Read the model definition and answer for the solid it produces. Units are mm, in the model's axes. A direction names the side the tool comes from. Coordinates: 2 decimals unless noted, no trailing zeros. Order: outer loops, then holes, each group sorted by start corner. A loop starts at its lowest first (then second) coordinate and runs counter-clockwise, first axis right, second up. Notation, with made-up numbers: (82.5, 85.25) -> (133.5, 85.25) arc R20 ccw to (133.5, 123.25) -> close; hole circle Ø4 at (-30.5, 59). An arc over 180 degrees is marked (long way). Use CSV: the item, a comma, the result in double quotes.
```python
from build123d import *

# Parameters (mm, degrees)
SKETCH1_R           = 10.16
BOSS_EXTRUDE1_DEPTH = 9.525
SKETCH2_W           = 20.151524415
SKETCH2_H           = 15.754496301
BOSS_EXTRUDE4_DEPTH = 3.175
BOSS_EXTRUDE5_DEPTH = 4.699
SKETCH4_W           = 11.36474419
SKETCH4_H           = 5.089940764
SKETCH4_W_2         = 11.314127359
BOSS_EXTRUDE6_DEPTH = 8.763
SKETCH5_W           = 19.083811061
SKETCH5_H           = 5.089940764
SKETCH5_W_2         = 19.185044725
BOSS_EXTRUDE7_DEPTH = 5.969


with BuildPart() as part:
    # Sketch1 → Boss-Extrude1 (new body)
    with BuildSketch(Plane.XY):
        Circle(SKETCH1_R)
    extrude(amount=-BOSS_EXTRUDE1_DEPTH)

    # Sketch2 → Boss-Extrude4 (add)
    with BuildSketch(Plane(origin=(0, 0, -9.525), x_dir=(-1, 0, 0), z_dir=(0, 0, -1))):
        with Locations((-0.084237792, 7.877248151)):
            Rectangle(SKETCH2_W, SKETCH2_H)
    extrude(amount=-BOSS_EXTRUDE4_DEPTH)

    # Sketch3 → Boss-Extrude5 (add)
    with BuildSketch(Plane(origin=(0, 15.754496301, 0), x_dir=(1, 0, 0), z_dir=(0, 1, 0))):
        Polygon((-9.991524415, 9.525), (-22.594029854, 9.525), (-22.594029854, 4.435059236), (23.166117059, 4.435059236), (23.166117059, 9.525), align=None)
    extrude(amount=BOSS_EXTRUDE5_DEPTH)

    # Sketch4 → Boss-Extrude6 (add)
    with BuildSketch(Plane(origin=(0, 20.453496301, 0), x_dir=(1, 0, 0), z_dir=(0, 1, 0))):
        with Locations((-16.911657759, 6.980029618)):
            Rectangle(SKETCH4_W, SKETCH4_H)
        with Locations((17.50905338, 6.980029618)):
            Rectangle(SKETCH4_W_2, SKETCH4_H)
    extrude(amount=BOSS_EXTRUDE6_DEPTH)

    # Sketch5 → Boss-Extrude7 (add)
    with BuildSketch(Plane(origin=(0, 29.216496301, 0), x_dir=(1, 0, 0), z_dir=(0, 1, 0))):
        with Locations((-13.052124324, 6.980029618)):
            Rectangle(SKETCH5_W, SKETCH5_H)
        with Locations((13.573594697, 6.980029618)):
            Rectangle(SKETCH5_W_2, SKETCH5_H)
    extrude(amount=BOSS_EXTRUDE7_DEPTH)


solid = part.part
```
Item 1: Straight lines are drawn through the part: line 1 along X through (y, z) = (28, -7); line 2 along Y through (x, z) = (-11, -9); line 3 along X through (y, z) = (5, -9). For each, find the intervals that lie inside material, in ascending order.
Return value:
line 1,"x = -22.59 to -11.23, 11.85 to 23.17"
line 2,"y = 15.75 to 20.45, 29.22 to 35.19"
line 3,"x = -9.99 to 10.16"
Item 2: A tool of negligible diameter and unlimited length cuts with its end or side. For faces 1 (the flat face through (3.981, 32, -7)), 2 (the flat face through (0, 11, -6.35)), 3 (the flat face through (8, 29.216, -7)), 4 (the flat face through (-9.992, 9, -8)), 5 (the flat face through (0, 19, -4.435)), from which of +Z, -Z, +X, -X, +Y, -Y can it reach the whole face along a straight path? Write none if from no direction.
Return value:
face 1,"+Z, -Z, +Y"
face 2,"+Z"
face 3,"+Z, -Z"
face 4,"+Z, -Z, -X"
face 5,"+Z, +X, -X, +Y"
Item 3: Find section A-A, the plane z = -5.5. Give the vertices of the cut face in (x, y).
Return value:
outline,"(-22.59, 15.75) -> (23.17, 15.75) -> (23.17, 35.19) -> (3.98, 35.19) -> (3.98, 29.22) -> (11.85, 29.22) -> (11.85, 20.45) -> (-11.23, 20.45) -> (-11.23, 29.22) -> (-3.51, 29.22) -> (-3.51, 35.19) -> (-22.59, 35.19) -> close; circle Ø20.32 at (0, 0)"
Item 4: Each of these flat-tipped pins is pushed along its axis until it touches: P1, Ø1.5, axis at x = 6.5, z = -7, coming from the -Y side; P2, Ø1, axis at y = 7, z = -7.5, coming from the -X side; P3, Ø6, axis at x = 9.5, y = 22, coming from the +Z side. Where does it stop, or does it pass through?
Return value:
P1,"stops at y = -8.38"
P2,"stops at x = -9.99"
P3,"stops at z = -4.44"
Item 5: Find section B-B, the plane y = 27. Give the vertices of the cut face in (x, z) (3 decimals).
Return value:
outline,"(-22.594, -9.525) -> (-11.229, -9.525) -> (-11.229, -4.435) -> (-22.594, -4.435) -> close; (11.852, -9.525) -> (23.166, -9.525) -> (23.166, -4.435) -> (11.852, -4.435) -> close"
Item 6: The mould has two halves that part along X. Classify faces 6 (the flat face through (-7, 29.216, -7)), 7 (the flat face through (0, 15.754, -6)), 8 (the flat face through (23.166, 25, -7)), 9 (the flat face through (-22.594, 25, -7)): +X half, -X half, draft (parallel to the pull), parting line (faces both ways), or undercut.
Return value:
face 6,"undercut"
face 7,"draft"
face 8,"+X half"
face 9,"-X half"
